Design review of the part shown in the three views and the two pictorial views. Dimensions are in mm from the part's minimum x, y and z. Coordinates: 2 decimals unless noted, no trailing zeros. Order: outer loops, then holes, each group sorted by start corner. A loop starts at its lowest first (then second) coordinate and runs counter-clockwise, first axis right, second up. Notation, with made-up numbers: (-25, 33) - (15, 33) arc R14 ccw to (15, 53) - close; hole circle Ø3 at (89.5, 59). An arc over 180 degrees is marked (long way). One line per item, written item: value. Start each with the question number.
(1) Consider section C-C on z = 4.9. Write out the cut boundary in (x, y) (3 decimals).
(2) To check wall thickness, follow line 1 along Y through (x, z) = (13.6, 0.1); line 2 along Y through (x, z) = (13.6, 5.1) (3 decimals); line 3 along Z through (x, y) = (21, 14.25). State the ranges of each line that lie inside material, in increasing order.
(3) Consider section D-D on z = 1.6. Write out the cut boundary in (x, y).
(4) Clearance check with flat-ended pins moving along their axes: pin 1 (2 mm diameter, centred on x = 15, y = 3, fed in from +Z); pin 2 (3 mm diameter, centred on x = 3.5, y = 15.5, fed in from -Z); pin 3 (10 mm diameter, centred on x = 14, y = 11, fed in from -Z). State where each tip first meets the part, or that it passes through.
(5) Mouldability with a two-part tool opening along X and no side actions: class the marked faces 1, 2 and 3 as released by +X, released by -X, zero draft, split by the parting line, or undercut.
(6) Consider section A-A on y = 13.6. Write out the cut boundary in (x, z) (3 decimals), then the cut area to 3 significant figures.
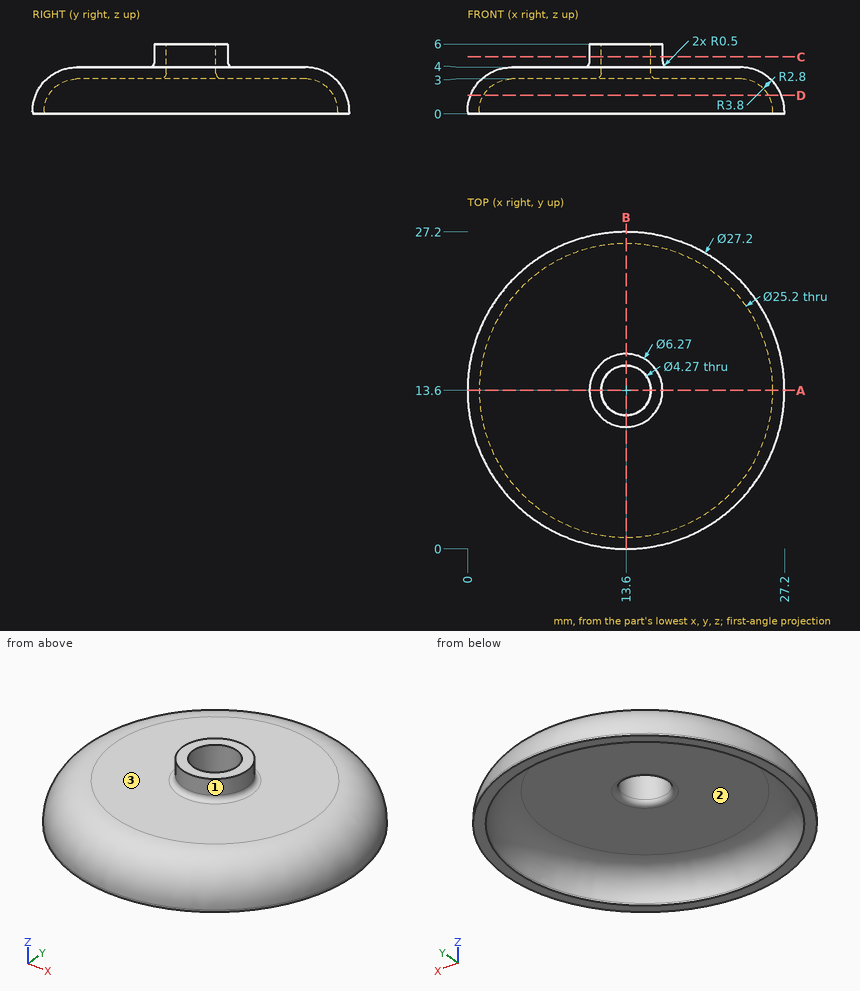
Geometry check:
1. outline: circle Ø6.27 at (13.6, 13.6); hole circle Ø4.27 at (13.6, 13.6)
2. line 1: y = 0 to 1, 26.2 to 27.2
2. line 2: y = 10.465 to 11.465, 15.735 to 16.735
2. line 3: z = 3 to 4
3. outline: circle Ø26.67 at (13.6, 13.6); hole circle Ø24.45 at (13.6, 13.6)
4. pin 1: stops at z = 4
4. pin 2: stops at z = 2.18
4. pin 3: stops at z = 3
5. face 1: split by the parting line
5. face 2: undercut
5. face 3: zero draft
6. outline: (0, 0) - (1, 0) - (1, 0.2) arc R2.8 cw to (3.8, 3) - (10.965, 3) arc R0.5 ccw to (11.465, 3.5) - (11.465, 6) - (10.465, 6) - (10.465, 4.5) arc R0.5 cw to (9.965, 4) - (3.8, 4) arc R3.8 ccw to (0, 0.2) - close; (15.735, 3.5) arc R0.5 ccw to (16.235, 3) - (23.4, 3) arc R2.8 cw to (26.2, 0.2) - (26.2, 0) - (27.2, 0) - (27.2, 0.2) arc R3.8 ccw to (23.4, 4) - (17.235, 4) arc R0.5 cw to (16.735, 4.5) - (16.735, 6) - (15.735, 6) - close
6. area: 30.1 mm^2
